Autodesk Inventor part; units mm, degrees
ref_plane "YZ Plane" through (0, 0, 0) normal (1, 0, 0) x (0, 1, 0)
ref_plane "XZ Plane" through (0, 0, 0) normal (0, 1, 0) x (-1, 0, 0)
ref_plane "XY Plane" through (0, 0, 0) normal (0, 0, 1) x (1, 0, 0)
sketch "Sketch1" plane through (0, 0, 0) normal (0, 0, 1) x (1, 0, 0)
  line L0 (0, 203.2) -> (0, 0)
  line L1 (0, 0) -> (-88.9, 0)
  line L2 (-196.2761, 150.608) -> (-196.2761, 107.3761)
  arc A0 (-196.2761, 107.3761) -> (-88.9, 0) centre (-88.9, 107.3761) ccw
  line L3 (-196.2761, 150.608) -> (0, 203.2)
  line L4 (0, -67.326) -> (0, 248.2877)
  dimension "d1" = 203.2
  dimension "d2" = 75
  dimension "d3" = 203.2
  dimension "d4" = 88.9
extrude "Extrusion1" add sketch "Sketch1" along normal mid plane 381
sketch "Sketch2" plane through (0, 0, 190.5) normal (1, 0, 0) x (0, 0, -1)
  circle A0 centre (88.9, 101.6) radius 88.9
  circle A1 centre (292.2878, 101.6) radius 88.9
  line L0 (381, 203.2) -> (0, 203.2)
  line L1 (0, 0) -> (0, 203.2)
  line L2 (381, 203.2) -> (381, 0)
  point P0 (190.5, 0)
  point P1 (0, 150.608)
  point P2 (366.6135, 150.374)
  point P3 (381, 0)
  point P4 (381, 107.3761)
  point P5 (0, 101.6)
  dimension "d7" = 177.8
  dimension "d8" = 177.8
  dimension "d16" = 101.6
  dimension "d17" = 101.6
extrude "Extrusion2" add sketch "Sketch2" along normal blind 767.08
properties part number "DMJ_Legs"
Work out the finished part from the listing and answer in its coordinate system (mm). A direction names the side the tool comes from. Give positions to 0.01 mm unless a question says otherwise; leave off trailing zeros. Order: outer loops, then holes, each group sorted by start corner. A loop starts at its lowest first (then second) coordinate and runs counter-clockwise, first axis right, second up. Notation, with made-up numbers: M -13,-4 L 46,-4 A21 cw 46,23 Z; hole C 77,-39 d1. An arc over 180 degrees is marked long. Return JSON: item names as keys, results as strings.
Q1. Find section B-B, the plane x = 218. Write down the section's boundary in (y, z).
Answer below:
{"outline": "C 101.6,-101.79 d177.8; C 101.6,101.6 d177.8"}
Q2. Find the intervals of material crossed by line 1 along Z through (x, y) = (201, 70); line 2 along Z through (x, y) = (-113, 123); line 3 along Z through (x, y) = (429.5, 48), in increasing order. Write a range as [from, to].
Answer below:
{"line 1": "z = [-184.88, -18.69], [18.51, 184.69]", "line 2": "z = [-190.5, 190.5]", "line 3": "z = [-172.71, -30.86], [30.68, 172.52]"}
Q3. Each of these flat-tipped pins is pushed along its axis until it touches: pin 1 (5 mm diameter, centred on x = 35, z = 37.5, fed in from +Y); pin 2 (12 mm diameter, centred on y = 80, z = -42, fed in from -X); pin 3 (2 mm diameter, centred on x = 523, y = 178, fed in from -Z). Where does it stop, or does it pass through?
Answer below:
{"pin 1": "stops at y = 165.7", "pin 2": "stops at x = -194.13", "pin 3": "stops at z = -148.88"}
Q4. The mould has two halves that part along Z. Classify faces 3 (the face through (378.17, 41.52, -36.26)), 4 (the face through (-163.99, 30.62, -2.67)), 5 (the face through (-78, 103, -190.5)): pulls with the +Z half, pulls with the -Z half, needs draft (parallel to the pull), parting line crosses it, or undercut.
Answer below:
{"face 3": "undercut", "face 4": "needs draft", "face 5": "pulls with the -Z half"}
Q5. Find section A-A, the plane z = 101.6. Write down the section's boundary in (x, y).
Answer below:
{"outline": "M -196.28,107.38 A107.38 ccw -88.9,0 L 0,0 L 0,12.7 L 767.08,12.7 L 767.08,190.5 L 0,190.5 L 0,203.2 L -196.28,150.61 Z"}
Q6. Find section D-D, the plane z = 50. Write down the section's boundary in (x, y).
Answer below:
{"outline": "M -196.28,107.38 A107.38 ccw -88.9,0 L 0,0 L 0,29.21 L 767.08,29.21 L 767.08,173.99 L 0,173.99 L 0,203.2 L -196.28,150.61 Z"}
Q7. Find section C-C, the plane y = 131. Write down the section's boundary in (x, z).
Answer below:
{"outline": "M -196.28,-190.5 L 0,-190.5 L 0,-185.69 L 767.08,-185.69 L 767.08,-17.89 L 0,-17.89 L 0,17.7 L 767.08,17.7 L 767.08,185.5 L 0,185.5 L 0,190.5 L -196.28,190.5 Z"}
Q8. Which of the six approach directions +Z, -Z, +X, -X, +Y, -Y give full straight-line access (tool end or side, diameter ignored) to faces 1 (the face through (378.17, 74.897, 16.805)), 2 (the face through (-99.512, 176.536, -2.667))?
Answer below:
{"face 1": "+X", "face 2": "+Z, -Z, -X, +Y"}
